Geometry: final body of the model. Coordinates: model frame, mm. A direction names the side the tool comes from. Give positions to 0.01 mm unless a question says otherwise; leave off trailing zeros. Write each loop counter-clockwise with the first axis right and the second up, starting at its lowest first coordinate (ties: lowest second). Pieces come first, ordered by that corner, then holes.
```python
from build123d import *

# Parameters (mm, degrees)
EXTRUDE_1_DEPTH = 25
SKETCH_2_R      = 0.6
EXTRUDE_2_DEPTH = 4


with BuildPart() as part:
    # 草图1 → 凸台-拉伸1 (new body)
    with BuildSketch(Plane.XY):
        Polygon((-11.6, 8.8), (-11.6, -8.2), (-10.4, -8.2), (-10.4, 0), (10.4, 0), (10.4, -8.2), (11.6, -8.2), (11.6, 8.8), (10.4, 8.8), (10.4, 2.5), (7.2, 2.5), (7.2, 8.8), (6, 8.8), (6, 1.2), (2.8, 1.2), (2.8, 8.8), (1.6, 8.8), (1.6, 2.5), (-1.6, 2.5), (-1.6, 8.8), (-2.8, 8.8), (-2.8, 1.2), (-6, 1.2), (-6, 8.8), (-7.2, 8.8), (-7.2, 2.5), (-10.4, 2.5), (-10.4, 8.8), align=None)
    extrude(amount=EXTRUDE_1_DEPTH)

    # 草图2 → 凸台-拉伸2 (add)
    with BuildSketch(Plane(origin=(0, 0, 0), x_dir=(-1, 0, 0), z_dir=(0, 0, -1))):
        with Locations(Location((-8.8, 1.8, 0), (0, 0, 180))):
            Circle(SKETCH_2_R)
        with Locations(Location((8.8, 1.8, 0), (0, 0, 180))):
            Circle(SKETCH_2_R)
    extrude(amount=EXTRUDE_2_DEPTH)


solid = part.part
```
Item 1: Section B-B, the plane y = 3. Return the cut outline in (x, z), plus the area to 3 significant figures.
Found:
outline: (-11.6, 0) - (-10.4, 0) - (-10.4, 25) - (-11.6, 25) - close; (-7.2, 0) - (-6, 0) - (-6, 25) - (-7.2, 25) - close; (-2.8, 0) - (-1.6, 0) - (-1.6, 25) - (-2.8, 25) - close; (1.6, 0) - (2.8, 0) - (2.8, 25) - (1.6, 25) - close; (6, 0) - (7.2, 0) - (7.2, 25) - (6, 25) - close; (10.4, 0) - (11.6, 0) - (11.6, 25) - (10.4, 25) - close
area: 180 mm2
Item 2: Section D-D, the plane x = -8.8. Return the cut outline in (y, z).
Found:
outline: (0, 0) - (1.2, 0) - (1.2, -4) - (2.4, -4) - (2.4, 0) - (2.5, 0) - (2.5, 25) - (0, 25) - close
Item 3: Section C-C, the plane z = -0.5. Return the cut outline in (x, y).
Found:
outline: circle Ø1.2 at (-8.8, 1.8); circle Ø1.2 at (8.8, 1.8)
Item 4: Pin query (flat end, axial travel): pin 1 Ø10.5 at (x, z) = (3.5, 8) entering from -Y; pin 2 Ø1 at (x, z) = (9, 6) entering from +Y; pin 3 Ø2.5 at (x, z) = (4.5, 14.5) entering from +Y. Return the tip coordinate at first contact, or that it passes through.
Found:
pin 1: stops at y = 0
pin 2: stops at y = 2.5
pin 3: stops at y = 1.2
Item 5: Reachability of faces 1 (the face through (-10.4, -4, 12)), 2 (the face through (-11, -8.2, 12)), 3 (the face through (-2.8, 5, 12)), 4 (the face through (-8.228, 1.62, -1.972)) from +Z, -Z, +X, -X, +Y, -Y: full face, straight path, thin tool, end or side. Return the list, or none.
Found:
face 1: +Z, -Z, -Y
face 2: +Z, -Z, +X, -X, -Y
face 3: +Z, -Z, +Y
face 4: -Z
Item 6: Line query: L1, parallel to X at y = 7.75, z = 11; L2, parallel to X at y = -1.75, z = 17.75; L3, parallel to Y at x = 10.25, z = 6.25. Output: solid intervals per line, ascending.
Found:
L1: x = -11.6 to -10.4, -7.2 to -6, -2.8 to -1.6, 1.6 to 2.8, 6 to 7.2, 10.4 to 11.6
L2: x = -11.6 to -10.4, 10.4 to 11.6
L3: y = 0 to 2.5
Item 7: Pull-direction query (X, two-part tool) for faces 5 (the face through (-11.6, 0, 12)), 6 (the face through (-2, 8.8, 12)), 7 (the face through (7.2, 6, 12)); classes: +X half, -X half, draft (parallel to the pull), parting line (faces both ways), or undercut.
Found:
face 5: -X half
face 6: draft
face 7: undercut
Item 8: Section A-A, the plane y = -4. Return the cut outline in (x, z).
Found:
outline: (-11.6, 0) - (-10.4, 0) - (-10.4, 25) - (-11.6, 25) - close; (10.4, 0) - (11.6, 0) - (11.6, 25) - (10.4, 25) - close
